For this review, take the finished solid that the model builds, in its own axes (mm). A direction names the side the tool comes from. Give positions to 0.01 mm unless a question says otherwise; leave off trailing zeros. Write each loop counter-clockwise with the first axis right and the second up, starting at its lowest first coordinate (ties: lowest second). Pieces come first, ordered by that corner, then holes.
from build123d import *

# Parameters (mm, degrees)
BOSS_EXTRUDE1_DEPTH     = 45
SKETCH3_OUTSIDE_W       = 59.222
SKETCH3_OUTSIDE_H       = 36.222
CUT_EXTRUDE1_DEPTH      = 18.5
CUT_EXTRUDE1_DEPTH_BACK = 18.5
CUT_EXTRUDE2_START      = -1.8
SKETCH5_OUTSIDE_W       = 48.562
SKETCH5_OUTSIDE_H       = 35.562
SKETCH5_OUTSIDE_W_2     = 20
SKETCH5_OUTSIDE_H_2     = 24.414034222
CUT_EXTRUDE2_DEPTH      = 39.604565841
F_2_CLEARANCE_HOLE1_D   = 2.4384
CUT_EXTRUDE3_START      = -2
SKETCH8_W               = 12
SKETCH8_H               = 64.371558748
CUT_EXTRUDE3_DEPTH      = 32.097482707


with BuildPart() as part:
    # Sketch1 → Boss-Extrude1 (new body)
    with BuildSketch(Plane.XY):
        with BuildLine():
            Line((-16.155172414, 2.502079991), (-6.068965517, 9.1742933))
            ThreePointArc((-6.068965517, 9.1742933), (0, 11), (6.068965517, 9.1742933))
            Line((6.068965517, 9.1742933), (16.155172414, 2.502079991))
            ThreePointArc((16.155172414, 2.502079991), (17.5, 0), (16.155172414, -2.502079991))
            Line((16.155172414, -2.502079991), (6.068965517, -9.1742933))
            ThreePointArc((6.068965517, -9.1742933), (0, -11), (-6.068965517, -9.1742933))
            Line((-6.068965517, -9.1742933), (-16.155172414, -2.502079991))
            ThreePointArc((-16.155172414, -2.502079991), (-17.5, 0), (-16.155172414, 2.502079991))
        make_face()
    extrude(amount=BOSS_EXTRUDE1_DEPTH)

    # Sketch3 outside → Cut-Extrude1 (cut, two sides)
    with BuildSketch(Plane(origin=(0, 0, 0), x_dir=(0, 0, -1), z_dir=(1, 0, 0))) as cut_extrude1_sk:
        with Locations((-22.5, 0)):
            Rectangle(SKETCH3_OUTSIDE_W, SKETCH3_OUTSIDE_H)
        Polygon((-25, 11), (-40.404565841, -11), (0, -11), (0, 11), align=None, mode=Mode.SUBTRACT)
    extrude(amount=CUT_EXTRUDE1_DEPTH, mode=Mode.SUBTRACT)
    extrude(cut_extrude1_sk.sketch, amount=-CUT_EXTRUDE1_DEPTH_BACK, mode=Mode.SUBTRACT)

    # Sketch5 outside → Cut-Extrude2 (cut, through all)
    with BuildSketch(Plane(origin=(0, 0, 0), x_dir=(-1, 0, 0), z_dir=(0, 0, -1)).offset(CUT_EXTRUDE2_START)):
        Rectangle(SKETCH5_OUTSIDE_W, SKETCH5_OUTSIDE_H)
        Rectangle(SKETCH5_OUTSIDE_W_2, SKETCH5_OUTSIDE_H_2, mode=Mode.SUBTRACT)
    extrude(amount=-CUT_EXTRUDE2_DEPTH, mode=Mode.SUBTRACT)

    # #2 Clearance Hole1 (through all)
    with Locations(Plane.XY.offset(1.8)):
        with Locations((14.5, 0), (-14.5, 0)):
            Hole(F_2_CLEARANCE_HOLE1_D / 2)

    # Sketch8 → Cut-Extrude3 (cut, through all)
    with BuildSketch(Plane(origin=(0, 15.365046972, 21.943561206), x_dir=(1, 0, 0), z_dir=(0, 0.573576436, 0.819152044)).offset(CUT_EXTRUDE3_START)):
        Rectangle(SKETCH8_W, SKETCH8_H)
    extrude(amount=-CUT_EXTRUDE3_DEPTH, mode=Mode.SUBTRACT)


solid = part.part
(1) The part is to be moulded in two halves that separate along X. For faces 1 (the flat face through (-8.8, -7.37, 19.29)), 2 (the flat face through (8.8, 7.37, 13.85)), 3 (the cylindrical face through (-13.28, 0.05, 0.89)), say which applies: +X half, -X half, draft (parallel to the pull), parting line (faces both ways), or undercut.
(2) Clearance check with flat-ended pins moving along their axes: pin 1 Ø3 at (x, y) = (4, -7.5) entering from +Z; pin 2 Ø1 at (x, y) = (11, 0) entering from +Z; pin 3 Ø5.5 at (y, z) = (0, 12.5) entering from +X; pin 4 Ø1.5 at (x, y) = (-14.5, 0) entering from -Z. State where each tip first meets the part, or that it passes through.
(3) We need section B-B (x = 14.5). Write out the cut boundary in (y, z), and give its area (3 significant figures).
(4) We need section C-C (y = 0). Write out the cut boundary in (x, z).
(5) We need section D-D (z = 32). Write out the cut boundary in (x, y).
(6) For L1, parallel to X at y = 0.75, z = 16; L2, parallel to Z at x = 12, y = 3; L3, parallel to Y at x = -14, z = 1, list the stretches that pass through material, from the lowest coordinate up.
(7) We need section A-A (z = 3). Write out the cut boundary in (x, y).
(8) Tool access review of faces 4 (the flat face through (11, 0, 0)), 5 (the flat face through (-0.084, 0.154, 30.153)), 6 (the flat face through (13, 0, 1.8)), 7 (the flat face through (-13, 0, 1.8)): name each direction out of +Z, -Z, +X, -X, +Y, -Y from which nothing blocks a thin tool from reaching the whole face with its end or side.
The answers:
1. face 1: -X half
1. face 2: +X half
1. face 3: undercut
2. pin 1: stops at z = 39
2. pin 2: stops at z = 1.8
2. pin 3: stops at x = 10
2. pin 4: passes through
3. outline: (-3.6, 0) - (-1.22, 0) - (-1.22, 1.8) - (-3.6, 1.8) - close; (1.22, 0) - (3.6, 0) - (3.6, 1.8) - (1.22, 1.8) - close
3. area: 8.56 mm2
4. outline: (-17.5, 0) - (-15.72, 0) - (-15.72, 1.8) - (-17.5, 1.8) - close; (-13.28, 0) - (-6, 0) - (-6, 30.26) - (6, 30.26) - (6, 0) - (13.28, 0) - (13.28, 1.8) - (10, 1.8) - (10, 32.7) - (-10, 32.7) - (-10, 1.8) - (-13.28, 1.8) - close; (15.72, 0) - (17.5, 0) - (17.5, 1.8) - (15.72, 1.8) - close
5. outline: (-10, -6.57) - (-6.07, -9.17) arc R11 ccw to (-6, -9.22) - (-6, -2.48) - (6, -2.48) - (6, -9.22) arc R11 ccw to (6.07, -9.17) - (10, -6.57) - (10, 1) - (-10, 1) - close
6. L1: x = -10 to -6, 6 to 10
6. L2: z = 0 to 1.8
6. L3: y = -3.93 to -1.11, 1.11 to 3.93
7. outline: (-10, -6.57) - (-6.07, -9.17) arc R11 ccw to (-6, -9.22) - (-6, 9.22) arc R11 ccw to (-6.07, 9.17) - (-10, 6.57) - close; (6, -9.22) arc R11 ccw to (6.07, -9.17) - (10, -6.57) - (10, 6.57) - (6.07, 9.17) arc R11 ccw to (6, 9.22) - close
8. face 4: -Z, +X, -X, +Y, -Y
8. face 5: -Z, -Y
8. face 6: +Z, +X, +Y, -Y
8. face 7: +Z, -X, +Y, -Y
